Autodesk Inventor part; units mm, degrees
ref_plane "YZ Plane" through (0, 0, 0) normal (1, 0, 0) x (0, 1, 0)
ref_plane "XZ Plane" through (0, 0, 0) normal (0, 1, 0) x (-1, 0, 0)
ref_plane "XY Plane" through (0, 0, 0) normal (0, 0, 1) x (1, 0, 0)
sketch "Sketch1" plane through (0, 0, 0) normal (1, 0, 0) x (0, 1, 0)
  line L0 (0, 0) -> (127, 0)
  line L1 (127, 0) -> (127, -25.4)
  line L2 (127, -25.4) -> (0, -25.4)
  line L3 (0, -25.4) -> (0, 0)
  line L4 (0, -6.35) -> (0, -19.05)
  line L5 (0, -6.35) -> (76.2, 0)
  line L6 (0, -19.05) -> (76.2, -25.4)
  dimension "d0" = 127
  dimension "d1" = 25.4
  dimension "d18" = 12.7
  dimension "d19" = 6.35
  dimension "d20" = 50.8
  dimension "d21" = 50.8
ref_plane "Work Plane1" through (44.5262, 0, 0) normal (1, 0, 0) x (0, 0, -1)
sketch "Sketch2" plane through (44.5262, 0, 0) normal (1, 0, 0) x (0, 0, -1)
  line L0 (0, 127) -> (0, 0)
  line L1 (0, 0) -> (25.4, 0)
  line L2 (25.4, 0) -> (25.4, 127)
  line L3 (25.4, 127) -> (0, 127)
  line L4 (0, 0) -> (25.4, 0)
  circle A0 centre (12.7, 0) radius 6.35
  dimension "d5" = 25.4
  dimension "d6" = 12.7
  dimension "d7" = 12.7
  dimension "d8" = 0
extrude "Extrusion2" add sketch "Sketch2" against normal blind 44.5262 contours A0 L1 | L1 A0
ref_plane "Work Plane2" through (44.5262, 0, 0) normal (1, 0, 0) x (0, 0, -1)
extrude "Extrusion3" add sketch "Sketch1" along normal blind 44.5262 contours L0 L1 L2 L6 L3 L5
sketch "Sketch4" plane through (0, 0, 0) normal (-1, 0, 0) x (0, 0, 1)
  arc A0 (-19.05, 0) -> (-6.35, 0) centre (-12.7, 0) ccw
  line L0 (0, 76.2) -> (-6.35, 0)
  line L1 (0, 127) -> (0, 76.2)
  line L2 (-25.4, 127) -> (0, 127)
  line L3 (-25.4, 76.2) -> (-25.4, 127)
  line L4 (-19.05, 0) -> (-25.4, 76.2)
  point P0 (0, 0)
hole "Hole2" at (0, 0, -12.7) direction (1, 0, 0) diameter 6.858 end through all
sketch "Sketch5" plane through (0, 0, 0) normal (-1, 0, 0) x (0, 0, 1)
  circle A0 centre (-12.7, 0) radius 3.429
  line L0 (0, 76.2) -> (-6.35, 0)
  line L1 (0, 127) -> (0, 76.2)
  line L2 (-25.4, 127) -> (0, 127)
  line L3 (-25.4, 76.2) -> (-25.4, 127)
  line L4 (-19.05, 0) -> (-25.4, 76.2)
  line L5 (-7.6835, 3.175) -> (43.1165, 3.175)
  line L6 (43.1165, 3.175) -> (43.1165, -3.175)
  line L7 (43.1165, -3.175) -> (-7.6835, -3.175)
  line L8 (-7.6835, -3.175) -> (-7.6835, 3.175)
  arc A1 (-19.05, 0) -> (-6.35, 0) centre (-12.7, 0) ccw
  point P0 (0, 0)
  dimension "d31" = 50.8
  dimension "d32" = 6.35
  dimension "d35" = 127
  dimension "d36" = 123.825
  dimension "d95" = 6.858
  dimension "d96" = 5.0165
extrude "Extrusion4" add sketch "Sketch5" against normal blind 44.5262 contours L5 L6 L7 A1 L0 | L0 A1 L7 L8 L5
sketch "Sketch8" plane through (0, 76.2, -25.4) normal (0, 0, -1) x (-1, 0, 0)
  line L0 (0, 0) -> (0, 50.8)
  line L1 (0, 50.8) -> (-44.5262, 50.8)
  line L2 (-44.5262, 0) -> (-44.5262, 50.8)
  line L3 (0, 0) -> (-44.5262, 0)
  line L4 (0, -76.2) -> (0, 0)
  line L5 (0, 0) -> (-44.5262, 0)
  line L6 (-44.5262, -76.2) -> (-44.5262, 0)
  line L7 (0, 50.8) -> (-44.5262, 50.8)
  line L8 (-39.7637, 50.8) -> (-4.7625, 50.8)
  line L9 (-4.7625, 50.8) -> (-4.7625, -98.425)
  line L10 (-4.7625, -98.425) -> (-39.7637, -98.425)
  line L11 (-39.7637, -98.425) -> (-39.7637, 50.8)
  line L12 (0, -76.2) -> (-44.5262, -76.2)
  point P0 (0, -76.2)
  dimension "d41" = 44.5262
  dimension "d43" = 35.0012
  dimension "d44" = 4.7625
  dimension "d45" = 149.225
extrude "Extrusion5" cut sketch "Sketch8" against normal blind 25.4 contours L9 L12 L11 L3 | L3 L11 L1 L9 | L9 L10 L11 L12
fillet "Fillet1" radius 3.175 2 edges at (39.7637, 0, 0) (4.7625, 0, 0)
fillet "Fillet2" radius 3.175 2 edges at (2.3812, 3.175, -6.0854) (42.1449, 3.175, -6.0854)
sketch "Sketch9" plane through (0, 0, 0) normal (-1, 0, 0) x (0, 0, 1)
  line L0 (0, 76.2) -> (-5.7989, 6.6137)
  line L1 (0, 127) -> (0, 76.2)
  line L2 (-25.4, 127) -> (0, 127)
  line L3 (-25.4, 76.2) -> (-25.4, 127)
  line L4 (-19.05, 0) -> (-25.4, 76.2)
  circle A0 centre (-12.7, 0) radius 3.429
  circle A1 centre (-12.7, 114.8637) radius 8
  line L5 (-19.6282, 118.8637) -> (-5.7718, 118.8637)
  line L6 (-5.7718, 118.8637) -> (-5.7718, 110.8637)
  line L7 (-5.7718, 110.8637) -> (-19.6282, 110.8637)
  line L8 (-19.6282, 110.8637) -> (-19.6282, 118.8637)
  arc A2 (-19.05, 0) -> (-7.2007, -3.175) centre (-12.7, 0) ccw
  line L9 (43.1165, -3.175) -> (-7.2007, -3.175)
  line L10 (43.1165, 3.175) -> (43.1165, -3.175)
  line L11 (-2.6348, 3.175) -> (43.1165, 3.175)
  arc A3 (-5.7989, 6.6137) -> (-2.6348, 3.175) centre (-2.6348, 6.35) ccw
  point P0 (0, 0)
  dimension "d50" = 16
  dimension "d51" = 25.4
  dimension "d52" = 12.7
  dimension "d53" = 8
  dimension "d54" = 4
hole "Hole3" at (0, 118.8637, -19.6282) at (0, 110.8637, -19.6282) at (0, 118.8637, -5.7718) at (0, 110.8637, -5.7718) direction (1, 0, 0) diameter 2.9718 depth 25.4 tip angle 118
sketch "Sketch10" plane through (44.5262, 0, 0) normal (1, 0, 0) x (0, 0, -1)
  line L0 (19.05, 0) -> (25.4, 76.2)
  line L1 (25.4, 76.2) -> (25.4, 127)
  line L2 (25.4, 127) -> (0, 127)
  line L3 (0, 127) -> (0, 76.2)
  line L4 (0, 76.2) -> (5.7989, 6.6137)
  circle A0 centre (12.7, 0) radius 3.429
  circle A1 centre (12.7, 113.546) radius 8
  line L5 (16.7, 106.6178) -> (8.7, 106.6178)
  line L6 (8.7, 106.6178) -> (8.7, 120.4742)
  line L7 (8.7, 120.4742) -> (16.7, 120.4742)
  line L8 (16.7, 120.4742) -> (16.7, 106.6178)
  arc A2 (7.2007, -3.175) -> (19.05, 0) centre (12.7, 0) ccw
  arc A3 (2.6348, 3.175) -> (5.7989, 6.6137) centre (2.6348, 6.35) ccw
  line L9 (2.6348, 3.175) -> (-43.1165, 3.175)
  line L10 (-43.1165, 3.175) -> (-43.1165, -3.175)
  line L11 (-43.1165, -3.175) -> (7.2007, -3.175)
  point P0 (0, 0)
  dimension "d62" = 16
  dimension "d63" = 25.4
  dimension "d64" = 12.7
  dimension "d65" = 8
  dimension "d66" = 4
hole "Hole4" at (44.5262, 106.6178, -16.7) at (44.5262, 106.6178, -8.7) at (44.5262, 120.4742, -8.7) at (44.5262, 120.4742, -16.7) direction (-1, 0, 0) diameter 2.9718 depth 25.4 tip angle 118
sketch "Sketch11" plane through (0, -3.175, -7.2007) normal (0, -1, 0) x (1, 0, 0)
  line L0 (4.7625, 0) -> (4.7625, 4.0257)
  arc A0 (7.9375, 7.2007) -> (4.7625, 4.0257) centre (7.9375, 4.0257) ccw
  line L1 (7.9375, 7.2007) -> (36.5887, 7.2007)
  arc A1 (39.7637, 4.0257) -> (36.5887, 7.2007) centre (36.5887, 4.0257) ccw
  line L2 (39.7637, 4.0257) -> (39.7637, 0)
  line L3 (44.5262, 50.3172) -> (44.5262, 0)
  line L4 (0, 50.3172) -> (44.5262, 50.3172)
  line L5 (0, 50.3172) -> (0, 0)
  line L6 (44.5262, 0) -> (39.7637, 0)
  line L7 (4.7625, 0) -> (0, 0)
  point P0 (0, 7.2007)
  point P1 (9.525, 42.1892)
  dimension "d74" = 8.128
  dimension "d75" = 44.5262
  dimension "d97" = 9.525
hole "Hole5" at (9.525, -3.175, 34.9885) direction (0, 1, 0) diameter 12.7 depth 3.175
sketch "Sketch12" plane through (44.5262, 0, 0) normal (1, 0, 0) x (0, 0, -1)
  circle A0 centre (8.7, 120.4742) radius 1.4859
  circle A1 centre (16.7, 106.6178) radius 1.4859
  circle A2 centre (8.7, 106.6178) radius 1.4859
  circle A3 centre (16.7, 120.4742) radius 1.4859
  line L0 (19.05, 0) -> (25.4, 76.2)
  line L1 (25.4, 76.2) -> (25.4, 127)
  line L2 (25.4, 127) -> (0, 127)
  line L3 (0, 127) -> (0, 76.2)
  line L4 (0, 76.2) -> (5.7989, 6.6137)
  circle A4 centre (12.7, 0) radius 3.429
  arc A5 (7.2007, -3.175) -> (19.05, 0) centre (12.7, 0) ccw
  arc A6 (2.6348, 3.175) -> (5.7989, 6.6137) centre (2.6348, 6.35) ccw
  line L5 (2.6348, 3.175) -> (-43.1165, 3.175)
  line L6 (-43.1165, 3.175) -> (-43.1165, -3.175)
  line L7 (-43.1165, -3.175) -> (7.2007, -3.175)
  point P0 (0, 0)
  point P1 (12.7, 113.546)
  dimension "d84" = 25.4
  dimension "d85" = 12.7
  dimension "d86" = 13.8564
  dimension "d87" = 6.9282
hole "Hole6" at (44.5262, 113.546, -12.7) direction (-1, 0, 0) diameter 6.35 end through all
equation "\"d19\" = -0.5 * d18 + 0.5 * d1"
equation "\"d21\" = d20"
equation "\"d7\" = 0.5 * d5"
equation "\"d36\" = d35 - 0.5 * d32"
equation "\"d44\" = -0.5 * d43 + 0.5 * d41"
equation "\"d52\" = 0.5 * d51"
equation "\"d54\" = 0.5 * d53"
equation "\"d64\" = 0.5 * d63"
equation "\"d66\" = 0.5 * d65"
properties part number "WheelIntakeMount3.0"
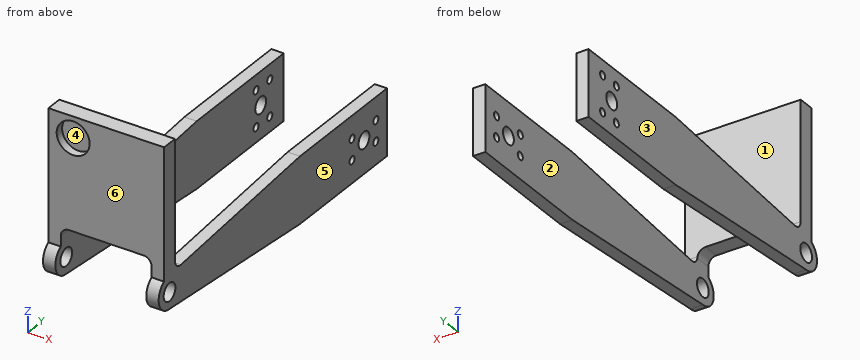
Check sheet for the modelled part. Datum: model origin and axes. Units: mm. Face numbers are marked on the shaded views. A direction names the side the tool comes from. Give positions to 0.01 mm unless a question says otherwise; leave off trailing zeros. Loops run counter-clockwise (first coordinate to the right, second up) from the corner with the lowest first, then second, coordinate; pieces in that order, holes last. Notation, with made-up numbers: M -10,41 L 39,41 A25 cw 39,72 Z; hole C 3.25,23.25 d9. An arc over 180 degrees is marked long. Answer as CSV lines item,"result".
Item 1: Scan lines: L1, parallel to Y at x = 40.85, z = -12.7; L2, parallel to X at y = 13, z = -19; L3, parallel to Z at x = 42, y = 0. Record each from-to range of solid material in increasing order.
Reply:
L1,"-6.35 to -3.43, 3.43 to 110.37, 116.72 to 127"
L2,"0 to 4.76, 39.76 to 44.53"
L3,"-19.05 to -16.13, -9.27 to 43.12"
Item 2: Depth check by flat-ended pin: pin 1 Ø3 at (x, z) = (25, 20.5) entering from +Y (3 decimals); pin 2 Ø1.4 at (x, y) = (43, 93.5) entering from +Z; pin 3 Ø8 at (x, z) = (39, 22.5) entering from -Y (3 decimals). Enter the tip coordinate at first touch or a pass-through.
Reply:
pin 1,"y = 3.175"
pin 2,"z = 0"
pin 3,"y = -3.175"
Item 3: Set-up check for the marked faces 4, 5 and 6: record each of +Z, -Z, +X, -X, +Y, -Y from which the full face is reachable in a straight line by a thin tool's end or side.
Reply:
face 4,"-Y"
face 5,"+Z, -Z, +X, +Y, -Y"
face 6,"+Z, +X, -X, -Y"
Item 4: Sectioned sample at C-C, the plane y = 57. Enter the section's corners in (x, z).
Reply:
outline,"M 0,-23.8 L 4.76,-23.8 L 4.76,-1.6 L 0,-1.6 Z; M 39.76,-23.8 L 44.53,-23.8 L 44.53,-1.6 L 39.76,-1.6 Z"
Item 5: Draft check along X on the marked faces 1, 2 and 3. Enter one of: pulls with the +X half, pulls with the -X half, needs draft (parallel to the pull), parting line crosses it, or undercut.
Reply:
face 1,"needs draft"
face 2,"undercut"
face 3,"pulls with the -X half"
Item 6: Sectioned sample at B-B, the plane z = -12.7. Enter the section's corners in (x, y), then the cut area to 3 significant figures.
Reply:
outline,"M 0,-6.35 L 4.76,-6.35 L 4.76,-3.43 L 0,-3.43 Z; M 0,3.43 L 4.76,3.43 L 4.76,110.37 L 0,110.37 Z; M 0,116.72 L 4.76,116.72 L 4.76,127 L 0,127 Z; M 39.76,-6.35 L 44.53,-6.35 L 44.53,-3.43 L 39.76,-3.43 Z; M 39.76,3.43 L 44.53,3.43 L 44.53,110.37 L 39.76,110.37 Z; M 39.76,116.72 L 44.53,116.72 L 44.53,127 L 39.76,127 Z"
area,"1,140 mm^2"
Item 7: Sectioned sample at A-A, the plane y = 97.5. Enter the section's corners in (x, z).
Reply:
outline,"M 0,-25.4 L 4.76,-25.4 L 4.76,0 L 0,0 Z; M 39.76,-25.4 L 44.53,-25.4 L 44.53,0 L 39.76,0 Z"
Item 8: Sectioned sample at D-D, the plane x = 35. Enter the section's corners in (y, z) (1 decimal).
Reply:
outline,"M -3.2,0 L 3.2,0 L 3.2,43.1 L -3.2,43.1 Z"
